```python
from build123d import *

# Parameters (mm, degrees)
F0_W           = 12
F0_H           = 8
F1_DEPTH       = 175
F1_DEPTH_BACK  = 175
F3_D           = 3.5
F3_CBORE_D     = 6
F3_CBORE_DEPTH = 3


with BuildPart() as f1:
    # F0 (on Front) → F1 (new body, two sides)
    with BuildSketch(Plane.XZ) as f1_sk:
        Rectangle(F0_W, F0_H)
    extrude(amount=F1_DEPTH)
    extrude(f1_sk.sketch, amount=-F1_DEPTH_BACK)

    # F3 (through all)
    with Locations(Plane.XY.offset(4)):
        with Locations((0, -162.5), (0, -137.5), (0, -112.5), (0, -87.5), (0, -62.5), (0, -37.5), (0, -12.5), (0, 12.5), (0, 37.5), (0, 62.5), (0, 87.5), (0, 112.5), (0, 137.5), (0, 162.5)):
            CounterBoreHole(F3_D / 2, F3_CBORE_D / 2, F3_CBORE_DEPTH)


solid = f1.part
```
Geometry check sheet. Reference: the model listing, model coordinates, mm. A direction names the side the tool comes from. Coordinates: 2 decimals unless noted, no trailing zeros.
Q1. Tool access check on faces 4 (the face through (0, -175, 0)), 5 (the face through (-0.391, -59.526, 2.521)). Record the directions out of +Z, -Z, +X, -X, +Y, -Y that give a thin tool (end or side, any length) a straight path to the whole face; none if there is none.
Reply:
face 4: +Z, -Z, +X, -X, -Y
face 5: +Z
Q2. Sectioned sample at A-A on z = -2. Give the number of separate pieces and of enclosed holes in the cut face, and give its area (3 significant figures).
Reply:
separate pieces: 1
enclosed holes: 14
area: 4,070 mm2
Q3. Thickness scan on probe 1 along X at (y, z) = (-162.5, 3.35); probe 2 along X at (y, z) = (113, -1.25). Record the ranges inside material, lowest first.
Reply:
probe 1: x = -6 to -3, 3 to 6
probe 2: x = -6 to -1.68, 1.68 to 6
Q4. Depth check by flat-ended pin: pin 1 Ø3 at (x, y) = (-1, -162.5) entering from +Z. Enter the tip coordinate at first touch or a pass-through.
Reply:
pin 1: stops at z = 1
Q5. Draft check along Y on faces 1 (the face through (0, -2, -4)), 2 (the face through (0, 175, 0)), 3 (the face through (2, -137, 1)). Enter one of: released by +Y, released by -Y, zero draft, split by the parting line, or undercut.
Reply:
face 1: zero draft
face 2: released by +Y
face 3: undercut
